Autodesk Inventor part; units mm, degrees
ref_plane "YZ Plane" through (0, 0, 0) normal (1, 0, 0) x (0, 1, 0)
ref_plane "XZ Plane" through (0, 0, 0) normal (0, 1, 0) x (-1, 0, 0)
ref_plane "XY Plane" through (0, 0, 0) normal (0, 0, 1) x (1, 0, 0)
ref_plane "Work Plane1" through (0, 41.8, 0) normal (0, 0, 1) x (1, 0, 0)
sketch "Sketch1" plane through (0, 41.8, 0) normal (0, 0, 1) x (1, 0, 0)
  line L0 (4, 0.3838) -> (4, 4) construction
  line L1 (4, 4) -> (-2, 4) construction
  arc A0 (-2, 4) -> (-4, 2) centre (-2, 2) ccw construction
  line L2 (-4, 2) -> (-4, -4) construction
  line L3 (-4, -4) -> (-0.3838, -4) construction
  arc A1 (45.8, 2) -> (43.8, 4) centre (43.8, 2) ccw construction
  line L4 (43.8, 4) -> (37.8, 4) construction
  line L5 (37.8, 4) -> (37.8, 0.3838) construction
  line L6 (42.1838, -4) -> (45.8, -4) construction
  line L7 (45.8, -4) -> (45.8, 2) construction
  line L8 (37.8, -42.1838) -> (37.8, -45.8) construction
  line L9 (37.8, -45.8) -> (43.8, -45.8) construction
  arc A2 (43.8, -45.8) -> (45.8, -43.8) centre (43.8, -43.8) ccw construction
  line L10 (45.8, -43.8) -> (45.8, -37.8) construction
  line L11 (45.8, -37.8) -> (42.1838, -37.8) construction
  line L12 (-0.3838, -37.8) -> (-4, -37.8) construction
  line L13 (-4, -37.8) -> (-4, -43.8) construction
  arc A3 (-4, -43.8) -> (-2, -45.8) centre (-2, -43.8) ccw construction
  line L14 (-2, -45.8) -> (4, -45.8) construction
  line L15 (4, -45.8) -> (4, -42.1838) construction
  line L16 (-2, 4) -> (43.8, 4)
  line L17 (45.8, 2) -> (45.8, -43.8)
  line L18 (43.8, -45.8) -> (-2, -45.8)
  line L19 (-4, -43.8) -> (-4, 2)
  line L20 (40.3, -37.8) -> (40.3, -4)
  line L21 (37.8, -1.5) -> (4, -1.5)
  line L22 (1.5, -4) -> (1.5, -37.8)
  line L23 (4, -40.3) -> (37.8, -40.3)
  line L24 (37.8, -40.3) -> (40.3, -37.8)
  line L25 (4, -40.3) -> (1.5, -37.8)
  line L26 (4, -1.5) -> (1.5, -4)
  line L27 (40.3, -4) -> (37.8, -1.5)
  arc A4 (45.8, 2) -> (43.8, 4) centre (43.8, 2) ccw
  arc A5 (43.8, -45.8) -> (45.8, -43.8) centre (43.8, -43.8) ccw
  arc A6 (-4, -43.8) -> (-2, -45.8) centre (-2, -43.8) ccw
  arc A7 (-2, 4) -> (-4, 2) centre (-2, 2) ccw
  circle A8 centre (1, -1) radius 1.4
  circle A9 centre (40.8, -1) radius 1.4
  circle A10 centre (40.8, -40.8) radius 1.4
  circle A11 centre (1, -40.8) radius 1.4
  circle A12 centre (20.9, -20.9) radius 19.4 construction
  line L28 (4, -4) -> (4, -37.8)
  line L29 (4, -37.8) -> (37.8, -37.8)
  line L30 (37.8, -37.8) -> (37.8, -4)
  line L31 (37.8, -4) -> (4, -4)
  arc A13 (39.5978, -40.386) -> (40.386, -39.5978) centre (40.9, -40.9) ccw
  line L32 (39.5978, -40.386) -> (37.8, -42.1838)
  line L33 (42.1838, -37.8) -> (40.386, -39.5978)
  arc A14 (1.414, -39.5978) -> (2.2022, -40.386) centre (0.9, -40.9) ccw
  line L34 (1.414, -39.5978) -> (-0.3838, -37.8)
  line L35 (4, -42.1838) -> (2.2022, -40.386)
  arc A15 (40.386, -2.2022) -> (39.5978, -1.414) centre (40.9, -0.9) ccw
  line L36 (40.386, -2.2022) -> (42.1838, -4)
  line L37 (37.8, 0.3838) -> (39.5978, -1.414)
  arc A16 (2.2022, -1.414) -> (1.414, -2.2022) centre (0.9, -0.9) ccw
  line L38 (2.2022, -1.414) -> (4, 0.3838)
  line L39 (-0.3838, -4) -> (1.414, -2.2022)
  point P0 (45.8, -45.8)
  point P1 (45.8, 4)
  point P2 (-4, -45.8)
  point P3 (40.3, -40.3)
  point P4 (40.3, -1.5)
  point P5 (1.5, -1.5)
  point P6 (1.5, -40.3)
  point P7 (40.8, -1)
  dimension "d55" = 2.8
  dimension "d56" = 2.8
  dimension "d57" = 2.8
  dimension "d58" = 2.8
  dimension "d34" = 49.8
  dimension "d35" = 49.8
  dimension "d36" = 5.5
  dimension "d37" = 2.5
  dimension "d38" = 2.5
  dimension "d39" = 2.5
  dimension "d40" = 2.5
  dimension "d41" = 2.5
  dimension "d42" = 2.5
  dimension "d43" = 2.5
  dimension "d44" = 2.5
  dimension "d45" = 2
  dimension "d46" = 5
  dimension "d47" = 5
  dimension "d48" = 5
  dimension "d49" = 5
  dimension "d50" = 5
  dimension "d51" = 5
  dimension "d52" = 0.5
  dimension "d53" = 5
  dimension "d54" = 5
  dimension "d90" = 8
extrude "Extrusion1" add sketch "Sketch1" along normal blind 8 contours L16 A4 L17 A5 L18 A6 L19 A7 | L24 L23 L25 L22 L26 L21 L27 L20 | A8 A16 | A9 A15 | A10 A13 | A14 A11
fillet "Fillet1" radius 2 8 edges at (20.9, -4, 8) (45.2142, -3.4142, 8) (45.8, 20.9, 8) (45.2142, 45.2142, 8) (20.9, 45.8, 8) (-3.4142, 45.2142, 8) (-4, 20.9, 8) (-3.4142, -3.4142, 8)
sketch "Sketch2" plane through (-2, -4, 0) normal (0, -1, 0) x (1, 0, 0)
  line L0 (43.8, -4.8712) -> (42.35, -4)
  line L1 (2, -4.8712) -> (0.55, -4)
  line L2 (-2, 0) -> (-2, 6) construction
  line L3 (45.8, 8) -> (0, 8) construction
  line L4 (47.8, 0) -> (47.8, 6) construction
  circle A0 centre (2.9, -36.9) radius 1.45
  line L5 (0, -41.8) -> (45.8, -41.8)
  point P0 (2, 0)
  point P1 (2.9, 3.1)
  point P2 (42.9, 3.1)
  dimension "d59" = 4.9
  dimension "d60" = 4.9
  dimension "d61" = 4.9
  dimension "d62" = 4.9
hole "Hole1" [suppressed]
sketch "Sketch3" plane through (0, 41.8, 8) normal (0, 0, 1) x (1, 0, 0)
  circle A0 centre (20.9, -20.9) radius 16.9 construction
  point P0 (0, -41.8)
sketch "Sketch4" plane through (0, 41.8, 8) normal (0, 0, 1) x (1, 0, 0)
  line L0 (37.8, -37.8) -> (37.8, -4)
  line L1 (37.8, -4) -> (4, -4)
  line L2 (4, -4) -> (4, -37.8)
  line L3 (4, -37.8) -> (37.8, -37.8)
  circle A0 centre (40.9, -0.9) radius 2.75
  circle A1 centre (0.9, -40.9) radius 2.75
  circle A2 centre (0.9, -0.9) radius 2.75
  circle A3 centre (40.9, -40.9) radius 2.75
  line L4 (43.8, 2) -> (-2, 2)
  line L5 (43.8, -43.8) -> (43.8, 2)
  line L6 (-2, -43.8) -> (43.8, -43.8)
  line L7 (-2, 2) -> (-2, -43.8)
hole "Hole2" at (40.9, 40.9, 8) at (40.9, 0.9, 8) at (0.9, 0.9, 8) at (0.9, 40.9, 8) direction (0, 0, -1) diameter 3.2 depth 12 tip angle 118 counterbore diameter 6 counterbore depth 2.5
chamfer "Chamfer2" distance 4.5 angle 45 2 edges at (4, 20.9, 0) (37.8, 20.9, 0)
sketch "Sketch6" plane through (-4, -2, 0) normal (-1, 0, 0) x (0, 0, 1)
  line L0 (0, -2) -> (6, -2) construction
  line L1 (8, 0) -> (8, 45.8) construction
  line L2 (0, 47.8) -> (6, 47.8) construction
  circle A0 centre (3.1, 42.9) radius 1.4 construction
  circle A1 centre (3.1, 2.9) radius 1.4 construction
  point P0 (0, 2)
  dimension "d63" = 2.8
  dimension "d64" = 2.8
  dimension "d65" = 4.9
  dimension "d66" = 4.9
  dimension "d67" = 4.9
  dimension "d68" = 4.9
hole "Hole3" [suppressed]
sketch "Sketch7" plane through (45.8, -2, 0) normal (1, 0, 0) x (0, 0, -1)
  circle A0 centre (-3.1, 42.9) radius 1.4
  circle A1 centre (-3.1, 2.9) radius 1.4
  point P0 (0, 2)
hole "Hole4" [suppressed]
sketch "Sketch8" plane through (-2, 45.8, 0) normal (0, 1, 0) x (1, 0, 0)
  circle A0 centre (2.9, -3.1) radius 1.45
  circle A1 centre (42.9, -3.1) radius 1.45
  point P0 (2, 0)
  point P1 (4.35, -3.1)
  point P2 (4.35, -3.1)
  point P3 (44.35, -3.1)
  point P4 (44.35, -3.1)
hole "Hole5" [suppressed]
sketch "Sketch9" plane through (37.8, 4, 8) normal (-1, 0, 0) x (0, 0, 1)
  line L0 (-8, 0) -> (-3.5, 0)
  line L1 (-3.5, 33.8) -> (-8, 33.8)
  line L2 (-3.5, 0) -> (-8, -4.5)
  line L3 (-8, 39.8) -> (-8, -6)
  line L4 (-3.5, 0) -> (2.864, 0) construction
  line L5 (-8, -4.5) -> (-8, 0)
  line L6 (-3.5, 33.8) -> (-8, 38.3)
  line L7 (-3.5, 33.8) -> (2.864, 33.8) construction
  line L8 (-8, 38.3) -> (-8, 33.8)
  line L9 (-8, 33.8) -> (-3.5, 33.8)
  point P0 (-8, -4)
  dimension "d91" = 135
  dimension "d92" = 135
extrude "Extrusion3" cut sketch "Sketch9" along normal up to surface (33.8 mm away)
sketch "Sketch13" plane through (0, 41.8, 0) normal (0, 0, -1) x (-1, 0, 0)
  line L0 (-37.8, -42.3) -> (-37.8, -37.8)
  line L1 (-37.8, -37.8) -> (-42.3, -37.8)
  line L2 (-42.3, -4) -> (-42.3, -37.8)
  line L3 (-42.3, -4) -> (-37.8, -4)
  line L4 (-37.8, -4) -> (-37.8, 0.5)
  line L5 (-37.8, 0.5) -> (-4, 0.5)
  line L6 (-4, 0.5) -> (-4, -4)
  line L7 (-4, -4) -> (0.5, -4)
  line L8 (0.5, -37.8) -> (0.5, -4)
  line L9 (0.5, -37.8) -> (-4, -37.8)
  line L10 (-4, -37.8) -> (-4, -42.3)
  line L11 (-4, -42.3) -> (-37.8, -42.3)
  circle A0 centre (-0.9, -40.9) radius 1.6
  circle A1 centre (-40.9, -0.9) radius 1.6
  circle A2 centre (-40.9, -40.9) radius 1.6
  circle A3 centre (-0.9, -0.9) radius 1.6
  line L12 (-45.8, 2) -> (-45.8, -43.8)
  arc A4 (-45.8, -43.8) -> (-43.8, -45.8) centre (-43.8, -43.8) ccw
  line L13 (-43.8, -45.8) -> (2, -45.8)
  arc A5 (2, -45.8) -> (4, -43.8) centre (2, -43.8) ccw
  line L14 (4, -43.8) -> (4, 2)
  arc A6 (4, 2) -> (2, 4) centre (2, 2) ccw
  line L15 (2, 4) -> (-43.8, 4)
  arc A7 (-43.8, 4) -> (-45.8, 2) centre (-43.8, 2) ccw
  point P0 (0, -41.8)
extrude "Extrusion5" cut sketch "Sketch13" against normal blind 4 contours L0 L1 L2 L3 L4 L5 L6 L7 L8 L9 L10 L11 | A7 L15 A6 L14 A5 L13 A4 L12
properties part number "10_Lid_1x1_v2_thin"
Geometry check sheet. Reference: the model listing, model coordinates, mm. A direction names the side the tool comes from. Give positions to 0.01 mm unless a question says otherwise; leave off trailing zeros. Order: outer loops, then holes, each group sorted by start corner. A loop starts at its lowest first (then second) coordinate and runs counter-clockwise, first axis right, second up. Notation, with made-up numbers: (24.25, -29) - (51.25, -29) arc R29 ccw to (51.25, -6) - close; hole circle Ø11 at (56.5, 75). An arc over 180 degrees is marked (long way). Answer in a Markdown table with one row per item. Add a question column.
Q1. Material ranges on probe 1 along Y at (x, z) = (40.9, 4.4); probe 2 along X at (y, z) = (40.9, 6), recorded low to high. Write a range as from..to.
Q2. Cross-section at D-D, the plane x = 40.9. Enter the section's corners in (y, z).
Q3. Cross-section at C-C, the plane z = 7.15. Enter the section's corners in (x, y).
Q4. Tool access check on faces 1 (the flat face through (37.8, 21, 6)), 2 (the cylindrical face through (0, 38.04, 6.73)), 3 (the flat face through (43, 21, 4)). Record the directions out of +Z, -Z, +X, -X, +Y, -Y that give a thin tool (end or side, any length) a straight path to the whole face; none if there is none.
Q5. Cross-section at A-A, the plane y = 20.5. Enter the section's corners in (x, z).
Q6. Mould release check, pull along Y, two halves, no side actions. Record for faces 4 (the cylindrical face through (-0.18, 42.08, 4.74)), 5 (the cylindrical face through (-3.4, -3.43, 4.99)), 6 (the flat face through (43.2, -1.4, 8)): pulls with the +Y half, pulls with the -Y half, needs draft (parallel to the pull), parting line crosses it, or undercut.
Q7. Gauge pin test, flat end, axial feed: pin 1 (3 mm diameter, centred on x = 41, y = 41, fed in from +Z). Record the tip position at first contact, or that the pin passes through.
Check values:
| question | item | result |
|---|---|---|
| 1 | probe 1 | y = -4..-0.7, 2.5..39.3, 42.5..45.8 |
| 1 | probe 2 | x = -4..-2.1, 3.9..37.9, 43.9..45.8 |
| 2 | outline | (-4, 4) - (-0.7, 4) - (-0.7, 5.5) - (-2.1, 5.5) - (-2.1, 8) arc R2 ccw to (-4, 6) - close; (2.5, 4) - (39.3, 4) - (39.3, 5.5) - (37.9, 5.5) - (37.9, 8) - (3.9, 8) - (3.9, 5.5) - (2.5, 5.5) - close; (42.5, 4) - (45.8, 4) - (45.8, 6) arc R2 ccw to (43.9, 8) - (43.9, 5.5) - (42.5, 5.5) - close |
| 3 | outline | (-3.64, -2) arc R1.64 ccw to (-2, -3.64) - (43.8, -3.64) arc R1.64 ccw to (45.44, -2) - (45.44, 43.8) arc R1.64 ccw to (43.8, 45.44) - (-2, 45.44) arc R1.64 ccw to (-3.64, 43.8) - close; hole circle Ø6 at (0.9, 0.9); hole circle Ø6 at (0.9, 40.9); hole (4, 4) - (37.8, 4) - (37.8, 37.8) - (4, 37.8) - close; hole circle Ø6 at (40.9, 0.9); hole circle Ø6 at (40.9, 40.9) |
| 4 | face 1 | +Z, -Z |
| 4 | face 2 | +Z |
| 4 | face 3 | -Z, +X, -X, +Y, -Y |
| 5 | outline | (-4, 4) - (3.5, 4) - (4, 4.5) - (4, 8) - (-2, 8) arc R2 ccw to (-4, 6) - close; (37.8, 4.5) - (38.3, 4) - (45.8, 4) - (45.8, 6) arc R2 ccw to (43.8, 8) - (37.8, 8) - close |
| 6 | face 4 | undercut |
| 6 | face 5 | pulls with the -Y half |
| 6 | face 6 | needs draft |
| 7 | pin 1 | stops at z = 5.5 |
